Geometry check sheet. Reference: the model listing, model coordinates, mm. Coordinates: 2 decimals unless noted, no trailing zeros. Write each loop counter-clockwise with the first axis right and the second up, starting at its lowest first coordinate (ties: lowest second). Pieces come first, ordered by that corner, then holes. Notation, with made-up numbers: M 9.5,-18.75 L 53.5,-18.75 A23 ccw 53.5,5.25 Z; hole C 85,39 d8. An arc over 180 degrees is marked long. Put each result on its own line as item: value. Start each with the question number.
1) Cross-section at A-A on y = -263. Record the cut outline in (x, z).
2) Scan lines: line 1 along X through (y, z) = (-629, 2); line 2 along Y through (x, z) = (-25.5, 1); line 3 along Y through (x, z) = (131, 4.6). Record each from-to range of solid material in increasing order.
3) Gauge pin test, flat ends, axial feed: pin 1 (6 mm diameter, centred on x = 280, y = -320.5, fed in from -Z); pin 2 (1 mm diameter, centred on y = -564, z = 3.5, fed in from -X); pin 3 (3 mm diameter, centred on y = 246, z = 2.5, fed in from -X); pin 4 (2 mm diameter, centred on x = 490, z = 4.5, fed in from -Y). Record the tip position at first contact, or that the pin passes through.
from build123d import *

# Parameters (mm, degrees)
F1_DEPTH = 5.08
F3_R     = 19.05


with BuildPart() as f1:
    # F0 (on Top) → F1 (new body)
    with BuildSketch(Plane.XY):
        with BuildLine():
            Line((330.2, -749.3), (330.2, 0))
            Line((330.2, 0), (774.7, 0))
            add(Edge.make_bspline(
                [(0, 469.9), (34.1164730489, 469.9), (385.0416966647, 476.161289739), (732.4479509774, 239.6232774633), (774.7, 0)],
                knots=[0, 0, 0, 0, 0.4227573718, 1, 1, 1, 1], degree=3))
            Line((0, 469.9), (0, 0))
            Line((0, 0), (0, -749.3))
            Line((0, -749.3), (330.2, -749.3))
        make_face()
    extrude(amount=F1_DEPTH)

    # F2: F1 across face


with BuildPart() as f1_1:
    add(f1.part)
    add(f1.part.mirror(Plane(origin=(0, -139.7, 2.54), x_dir=(0, -1, 0), z_dir=(-1, 0, 0))))

    # F3
    f3_edges = [f1_1.edges().sort_by_distance(p)[0] for p in [
        (-774.7, 0, 2.54),
        (774.7, 0, 2.54),
    ]]
    fillet(f3_edges, radius=F3_R)


solid = f1_1.part
Answer key:
1. outline: M -330.2,0 L 330.2,0 L 330.2,5.08 L -330.2,5.08 Z
2. line 1: x = -330.2 to 330.2
2. line 2: y = -749.3 to 469.91
2. line 3: y = -749.3 to 465.47
3. pin 1: stops at z = 0
3. pin 2: stops at x = -330.2
3. pin 3: stops at x = -653.53
3. pin 4: stops at y = 0
